Could you check a few things on this model? Use its own coordinates, in mm. Give positions to 0.01 mm unless a question says otherwise; leave off trailing zeros. Order: outer loops, then holes, each group sorted by start corner. A loop starts at its lowest first (then second) coordinate and runs counter-clockwise, first axis right, second up. Notation, with made-up numbers: M 51,82 L 96,82 A10 cw 96,88 Z; hole C -21,15.25 d4. An arc over 180 degrees is marked long. Use a Markdown table: item, result. Add a question column.
Item 1: Suppose I cut it at C-C on x = 36.5. Write out the boundary of the cut face in (y, z).
Item 2: Suppose I cut it at B-B on y = 0.5. Write out the boundary of the cut face in (x, z), plus the area to 3 significant figures.
Item 3: I'm going to push flat-ended pins straight in: pin 1 Ø5 at (x, z) = (36.5, 3.55) entering from -Y; pin 2 Ø1 at (y, z) = (0.5, 6) entering from -X; pin 3 Ø1 at (y, z) = (0.5, 10) entering from +X. Where does each tip first touch, or does it pass through?
Item 4: Suppose I cut it at A-A on z = 6.2. Write out the boundary of the cut face in (x, y), plus the area to 3 significant figures.
Item 5: Suppose I cut it at D-D on z = 0. Write out the boundary of the cut face in (x, y), plus the area to 3 significant figures.
Item 6: If I drill on L1, parallel to Z at x = 0, y = 1.35; L2, parallel to X at y = 1.45, z = 6.2; L3, parallel to Z at x = 57.5, y = 1.05, over which ranges is the centre line in solid material (lowest first)? Write a range as from..to.
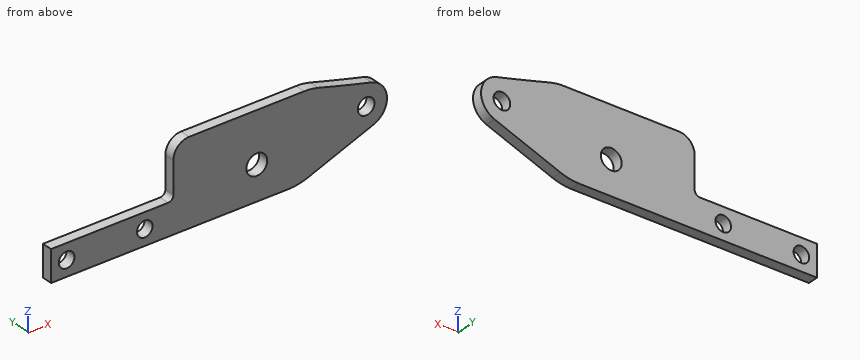
from build123d import *

# Parameters (mm, degrees)
SKETCH_2_R          = 1.5
SKETCH_2_R_2        = 1.6
EXTRUDE_2_DEPTH     = 2
FILLET_1_R          = 1
FILLET_2_R          = 10
SKETCH_3_R          = 2
CUT_EXTRUDE_1_DEPTH = 3


with BuildPart() as part:
    # 草图2 → 凸台-拉伸2 (new body)
    with BuildSketch(Plane(origin=(0, 0, 0), x_dir=(1, 0, 0), z_dir=(0, 1, 0))):
        with BuildLine():
            Line((44.5, 3), (-3, 3))
            Line((-3, 3), (-3, -3))
            Line((-3, -3), (20.5, -3))
            Line((20.5, -3), (20.5, -10.2))
            ThreePointArc((20.5, -10.2), (21.378679656, -12.321320344), (23.5, -13.2))
            Line((23.5, -13.2), (45.594157258, -13.2))
            ThreePointArc((45.594157258, -13.2), (46.977327515, -13.10388005), (48.333907722, -12.817368008))
            ThreePointArc((48.333907722, -12.817368008), (53.401969584, -11.411447703), (58.489004431, -10.075805753))
            ThreePointArc((58.489004431, -10.075805753), (61.493712967, -6.424180145), (58.916547929, -2.459225753))
            Line((58.916547929, -2.459225753), (44.5, 3))
        make_face()
        Circle(SKETCH_2_R, mode=Mode.SUBTRACT)
        with Locations((15, 0)):
            Circle(SKETCH_2_R, mode=Mode.SUBTRACT)
        with Locations((57.5, -6.2)):
            Circle(SKETCH_2_R_2, mode=Mode.SUBTRACT)
    extrude(amount=EXTRUDE_2_DEPTH)

    # 圆角1
    fillet_1_edges = [part.edges().sort_by_distance(p)[0] for p in [
        (20.5, 1, 3),
    ]]
    fillet(fillet_1_edges, radius=FILLET_1_R)

    # 圆角2
    fillet_2_edges = [part.edges().sort_by_distance(p)[0] for p in [
        (44.5, 1, -3),
    ]]
    fillet(fillet_2_edges, radius=FILLET_2_R)

    # 草图3 → 切除-拉伸1 (cut, through all)
    with BuildSketch(Plane(origin=(0, 2, 0), x_dir=(1, 0, 0), z_dir=(0, 1, 0))):
        with Locations((36.5, -3.55)):
            Circle(SKETCH_3_R)
    extrude(amount=-CUT_EXTRUDE_1_DEPTH, mode=Mode.SUBTRACT)


solid = part.part
Findings below:
| question | item | result |
|---|---|---|
| 1 | outline | M 0,-3 L 2,-3 L 2,1.55 L 0,1.55 Z; M 0,5.55 L 2,5.55 L 2,13.2 L 0,13.2 Z |
| 2 | outline | M -3,-3 L 42.67,-3 A10 ccw 46.21,-2.35 L 58.92,2.46 A4 ccw 58.49,10.08 A380 cw 48.33,12.82 A10 ccw 45.59,13.2 L 23.5,13.2 A3 ccw 20.5,10.2 L 20.5,4 A1 cw 19.5,3 L -3,3 Z; hole C 0,0 d3; hole C 15,0 d3; hole C 36.5,3.55 d4; hole C 57.5,6.2 d3.2 |
| 2 | area | 682 mm^2 |
| 3 | pin 1 | stops at y = 0 |
| 3 | pin 2 | stops at x = 20.5 |
| 3 | pin 3 | stops at x = 59.76 |
| 4 | outline | M 20.5,0 L 55.9,0 L 55.9,2 L 20.5,2 Z; M 59.1,0 L 61.5,0 L 61.5,2 L 59.1,2 Z |
| 4 | area | 75.6 mm^2 |
| 5 | outline | M -3,0 L -1.5,0 L -1.5,2 L -3,2 Z; M 1.5,0 L 13.5,0 L 13.5,2 L 1.5,2 Z; M 16.5,0 L 52.42,0 L 52.42,2 L 16.5,2 Z |
| 5 | area | 98.8 mm^2 |
| 6 | L1 | z = -3..-1.5, 1.5..3 |
| 6 | L2 | x = 20.5..55.9, 59.1..61.5 |
| 6 | L3 | z = 1.92..4.6, 7.8..10.33 |
